```python
from build123d import *

# Parameters (mm, degrees)
F1_DEPTH = 10.033
F3_DEPTH = 76.2
F5_DEPTH = 76.2


with BuildPart() as f1:
    # F0 (on Right) → F1 (new body, symmetric)
    with BuildSketch(Plane.YZ):
        Polygon((16.51, -4.445), (25.4, 4.445), (-16.51, 4.445), (-25.4, -4.445), align=None)
    extrude(amount=F1_DEPTH, both=True)

    # F2 (on Front) → F3 (cut, symmetric)
    with BuildSketch(Plane.XZ):
        Polygon((3.5941, 7.676974), (-3.5941, 7.676974), (-3.5941, 2.5908), (-6.00075, 2.5908), (-6.00075, 0.3683), (6.00075, 0.3683), (6.00075, 2.5908), (3.5941, 2.5908), align=None)
    extrude(amount=F3_DEPTH, both=True, mode=Mode.SUBTRACT)

    # F4 (on Front) → F5 (cut, symmetric)
    with BuildSketch(Plane.XZ):
        Polygon((-6.858, -1.905), (-5.588, -4.445), (5.588, -4.445), (6.858, -1.905), align=None)
    extrude(amount=F5_DEPTH, both=True, mode=Mode.SUBTRACT)


solid = f1.part
```
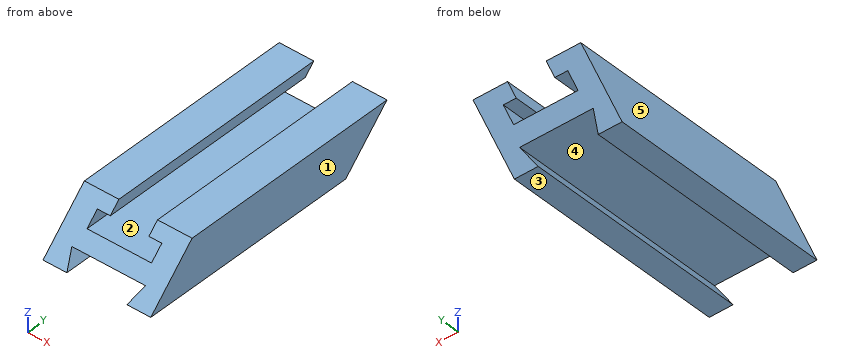
Geometry: final body of the model. Coordinates: model frame, mm. Face numbers are marked on the shaded views. A direction names the side the tool comes from. Coordinates: 2 decimals unless noted, no trailing zeros. Order: outer loops, then holes, each group sorted by start corner. A loop starts at its lowest first (then second) coordinate and runs counter-clockwise, first axis right, second up. Notation, with made-up numbers: (-6.75, 14.5) - (24.25, 14.5) arc R19 cw to (24.25, 31.5) - close; hole circle Ø3 at (39, 24). An arc over 180 degrees is marked (long way). Write each question's results on one line, items separated by ' | '.
(1) Section query A-A, the plane x = 5. Return the cut outline in (y, z) (3 decimals), plus the area to 3 significant figures.
Values found:
outline: (-22.86, -1.905) - (19.05, -1.905) - (21.323, 0.368) - (-20.587, 0.368) - close; (-18.364, 2.591) - (23.546, 2.591) - (25.4, 4.445) - (-16.51, 4.445) - close | area: 173 mm²
(2) Section query C-C, the plane y = -15. Return the cut outline in (x, z) (3 decimals), plus the area to 3 significant figures.
Values found:
outline: (-10.033, -4.445) - (-5.588, -4.445) - (-6.858, -1.905) - (6.858, -1.905) - (5.588, -4.445) - (10.033, -4.445) - (10.033, 4.445) - (3.594, 4.445) - (3.594, 2.591) - (6.001, 2.591) - (6.001, 0.368) - (-6.001, 0.368) - (-6.001, 2.591) - (-3.594, 2.591) - (-3.594, 4.445) - (-10.033, 4.445) - close | area: 107 mm²
(3) Section query B-B, the plane z = 1.5. Return the cut outline in (x, y) (3 decimals).
Values found:
outline: (-10.033, -19.455) - (-6.001, -19.455) - (-6.001, 22.455) - (-10.033, 22.455) - close; (6.001, -19.455) - (10.033, -19.455) - (10.033, 22.455) - (6.001, 22.455) - close
(4) Line query: line 1 (X direction, y = 19, z = 2.75); line 2 (X direction, y = -14, z = 0.5); line 3 (Z direction, x = 4.75, y = 1) (3 decimals). Output: solid intervals per line, ascending. Write a range as [from, to].
Values found:
line 1: x = [-10.03, -3.59], [3.59, 10.03] | line 2: x = [-10.03, -6], [6, 10.03] | line 3: z = [-1.905, 0.368], [2.591, 4.445]
(5) Section query D-D, the plane x = -0.75. Return the cut outline in (y, z) (3 decimals), plus the area to 3 significant figures.
Values found:
outline: (-22.86, -1.905) - (19.05, -1.905) - (21.323, 0.368) - (-20.587, 0.368) - close | area: 95.3 mm²
(6) First-contact query: pin 1 Ø4 at (x, y) = (2, 20) entering from -Z (3 decimals); pin 2 Ø6 at (x, y) = (-1, 3) entering from +Z (3 decimals); pin 3 Ø2 at (x, y) = (-2.5, 12) entering from +Z. Flat tips, straight axial feed; report the tip coordinate or a pass-through.
Values found:
pin 1: stops at z = -1.905 | pin 2: stops at z = 4.445 | pin 3: stops at z = 0.37
(7) Set-up query: the marked faces 4 and 5. Return all of +Z, -Z, +X, -X, +Y, -Y with unobstructed straight access to the full face (end or side cutting, diameter ignored); none if empty.
Values found:
face 4: +Y, -Y | face 5: +Z, -Z, -X, +Y, -Y
(8) Mould query, pull axis X, two halves, no side actions, for the marked faces 1, 2 and 3. Classes: +X half, -X half, draft (parallel to the pull), parting line (faces both ways), or undercut.
Values found:
face 1: +X half | face 2: undercut | face 3: draft
